Source: CAD feature listing. Evaluate the final solid. Frame: model axes, mm. Face numbers are marked on the shaded views. Coordinates: 2 decimals unless noted, no trailing zeros. Write each loop counter-clockwise with the first axis right and the second up, starting at its lowest first coordinate (ties: lowest second). Pieces come first, ordered by that corner, then holes. Notation, with made-up numbers: (-32, -12.75) - (27, -12.75) arc R12 cw to (27, 0.25) - close; hole circle Ø5 at (-18.5, 87.5). An arc over 180 degrees is marked (long way). One line per question, with ' | ' between items.
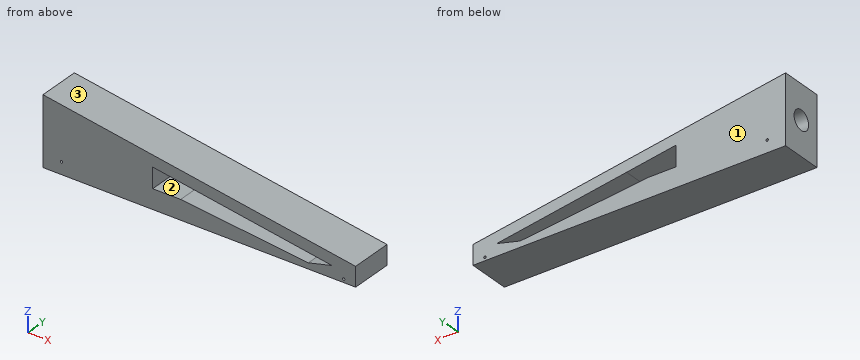
from build123d import *

# Parameters (mm, degrees)
F1_DEPTH  = 41.275
F2_R      = 9.525
F3_DEPTH  = 50.8
F5_DEPTH  = 45.72
F7_DEPTH  = 60.96
F8_R      = 1.190625
F9_DEPTH  = 63.5
F10_R     = 1.190625
F11_DEPTH = 63.5


with BuildPart() as f1:
    # F0 (on Front) → F1 (new body)
    with BuildSketch(Plane.XZ):
        Polygon((-152.966577, 66.675), (-152.966577, 0), (151.833423, 0), (151.833423, 19.05), align=None)
    extrude(amount=F1_DEPTH)

    # F2 (on face) → F3 (cut)
    with BuildSketch(Plane(origin=(-152.966577, 0, 0), x_dir=(0, -1, 0), z_dir=(-1, 0, 0))):
        with Locations((20.6375, 33.3375)):
            Circle(F2_R)
    extrude(amount=-F3_DEPTH, mode=Mode.SUBTRACT)

    # F4 (on face) → F5 (cut)
    with BuildSketch(Plane.XZ.offset(41.275)):
        Polygon((105.732426, 5.715), (128.846437, 11.557001), (2.083721, 31.363675), (-18.727573, 19.05), align=None)
    extrude(amount=-F5_DEPTH, mode=Mode.SUBTRACT)

    # F6 (on face) → F7 (cut)
    with BuildSketch(Plane.XZ.offset(41.275)):
        Polygon((-18.727573, 19.05), (-46.036839, 38.882513), (-46.036839, 19.05), align=None)
        Polygon((-18.727573, 19.05), (2.083721, 31.363675), (-46.036839, 38.882513), align=None)
    extrude(amount=-F7_DEPTH, mode=Mode.SUBTRACT)

    # F8 (on face) → F9 (cut)
    with BuildSketch(Plane(origin=(0, 0, 0), x_dir=(-1, 0, 0), z_dir=(0, 1, 0))):
        with Locations((134.939879, 11.659147)):
            Circle(F8_R)
    extrude(amount=-F9_DEPTH, mode=Mode.SUBTRACT)

    # F10 (on face) → F11 (cut)
    with BuildSketch(Plane(origin=(0, 0, 0), x_dir=(-1, 0, 0), z_dir=(0, 1, 0))):
        with Locations((-140.181614, 3.221456)):
            Circle(F10_R)
    extrude(amount=-F11_DEPTH, mode=Mode.SUBTRACT)


solid = f1.part
Item 1: Cut plane D-D on x = -4.5. Return loops of the section in (y, z) (3 decimals).
Check sheet entries:
outline: (-41.275, 0) - (0, 0) - (0, 17.526) - (-41.275, 17.526) - close; (-41.275, 32.392) - (0, 32.392) - (0, 43.477) - (-41.275, 43.477) - close
Item 2: Ray query, line 1 along X through (y, z) = (-6, 3.5); line 2 along Z through (x, y) = (-15.5, -16); line 3 along Z through (x, y) = (17.5, -4). Return the intervals inside material, ascending. Write a range as [from, to].
Check sheet entries:
line 1: [-152.97, 139.02], [141.34, 151.83] | line 2: [0, 18.7], [34.11, 45.2] | line 3: [0, 15.17], [28.95, 40.04]
Item 3: Cut plane B-B on y = -23. State how many separate pieces and enclosed holes the cut face has, and give its area (3 significant figures).
Check sheet entries:
separate pieces: 1 | enclosed holes: 3 | area: 9,970 mm²
Item 4: Mould query, pull axis X, two halves, no side actions, for the marked faces 1, 2 and 3. Classes: pulls with the +X half, pulls with the -X half, needs draft (parallel to the pull), parting line crosses it, or undercut.
Check sheet entries:
face 1: needs draft | face 2: undercut | face 3: pulls with the +X half
Item 5: Cut plane A-A on x = 62.5. Return loops of the section in (y, z) (3 decimals).
Check sheet entries:
outline: (-41.275, 0) - (0, 0) - (0, 10.347) - (-41.275, 10.347) - close; (-41.275, 21.924) - (0, 21.924) - (0, 33.008) - (-41.275, 33.008) - close
Item 6: Pin query (flat end, axial travel): pin 1 Ø13.5 at (x, y) = (-35, -11) entering from +Z; pin 2 Ø1.5 at (x, y) = (-47, -9.5) entering from +Z; pin 3 Ø1.4 at (x, z) = (-134.94, 11.66) entering from -Y; pin 4 Ø12 at (x, y) = (69, -6.5) entering from +Z. Return the tip coordinate at first contact, or that it passes through.
Check sheet entries:
pin 1: z = 49.3 | pin 2: z = 50.23 | pin 3: through | pin 4: z = 32.93
